The model under review builds one solid part; all positions refer to its coordinate system, in mm. A direction names the side the tool comes from. Coordinates: 2 decimals unless noted, no trailing zeros. Write each loop counter-clockwise with the first axis right and the second up, starting at its lowest first coordinate (ties: lowest second). Pieces come first, ordered by that corner, then holes. Notation, with made-up numbers: M 44,76 L 51,76 A12 cw 51,86 Z; hole C 48,52.25 d5. An arc over 180 degrees is marked long. Answer as CSV lines item,"result". Start each with the question number.
from build123d import *

# Parameters (mm, degrees)
F0_W        = 67.24
F0_H        = 39
F1_DEPTH    = 1.5
F2_T1_DEPTH = 49.2867319519
F3_T1_DEPTH = 73.5267319519
F3_T3_DEPTH = 43.5142834408
F4_R        = 1
F5_DEPTH    = 2
F6_W        = 16
F6_H        = 3.0143252599
F7_DEPTH    = 2


# Not quite as in the source:
# - a fillet or chamfer that OpenCascade refuses, or shapes differently, is made with other operations: its cross-section is extruded or revolved along the edge and cut away or added


with BuildPart() as f1:
    # F0 (on Top) → F1 (new body)
    with BuildSketch(Plane.XY):
        with Locations((12.5632099807, -23.9098862686)):
            Rectangle(F0_W, F0_H)
    extrude(amount=F1_DEPTH)

    # F2: chamfer of 2 on 2 edges, made by hand

    # F2_s2 → F2_t1 (cut)
    with BuildSketch(Plane.XZ.offset(-0.7334797074)):
        Polygon((46.1832099807, -0.5), (44.1832099807, 1.5), (46.1832099807, 1.5), align=None)
        Polygon((-21.0567900193, -0.5), (-19.0567900193, 1.5), (-21.0567900193, 1.5), align=None)
    extrude(amount=F2_T1_DEPTH, mode=Mode.SUBTRACT)

    # F3: chamfer of 2 on 4 edges, made by hand

    # F3_s2 → F3_t1 (cut)
    with BuildSketch(Plane.YZ.offset(-24.2001559952)):
        Polygon((-4.4098862686, -0.5), (-6.4098862686, 1.5), (-4.4098862686, 1.5), align=None)
        Polygon((-41.4098862686, 1.5), (-43.4098862686, -0.5), (-43.4098862686, 1.5), align=None)
    extrude(amount=F3_T1_DEPTH, mode=Mode.SUBTRACT)

    # F3_s4 → F3_t3 (cut)
    with BuildSketch(Plane.XZ.offset(2.1527445482)):
        Polygon((43.354782856, 1.5), (44.7689964183, 0.9142135624), (44.1832099807, 1.5), align=None)
        Polygon((-19.6425764569, 0.9142135624), (-18.2283628946, 1.5), (-19.0567900193, 1.5), align=None)
    extrude(amount=F3_T3_DEPTH, mode=Mode.SUBTRACT)

    # F4 (on face) → F5 (cut)
    with BuildSketch(Plane.XY.offset(1.5)):
        with Locations((43.1832099807, -40.4098862686)):
            Circle(F4_R)
        with Locations((43.1832099807, -7.4098862686)):
            Circle(F4_R)
        with Locations((-18.0567900193, -40.4098862686)):
            Circle(F4_R)
        with Locations((-18.0567900193, -7.4098862686)):
            Circle(F4_R)
    extrude(amount=-F5_DEPTH, mode=Mode.SUBTRACT)

    # F6 (on face) → F7 (cut)
    with BuildSketch(Plane.XY.offset(1.5)):
        with Locations((12.6832099807, -10.7027236386)):
            Rectangle(F6_W, F6_H)
    extrude(amount=-F7_DEPTH, mode=Mode.SUBTRACT)


solid = f1.part
1) Clearance check with flat-ended pins moving along their axes: pin 1 Ø0.8 at (x, z) = (9.5, 0.5) entering from -Y; pin 2 Ø2.5 at (x, y) = (-18.06, -40.41) entering from +Z. State where each tip first meets the part, or that it passes through.
2) To check wall thickness, follow line 1 (Y direction, x = 42.5, z = 0.15); line 2 (X direction, y = -7.5, z = 0.8); line 3 (X direction, y = -8, z = 0.5). State the ranges of each line that lie inside material, in increasing order. Write a range as [from, to].
3) Take a section at C-C on y = -24. Give the boundary of the cut face in (x, z).
4) Mouldability with a two-part tool opening along Y and no side actions: class faces 1 (the flat face through (-18.95, -23.66, 1.2)), 2 (the flat face through (12.1, -42.15, 0.76)), 3 (the cylindrical face through (-17.103, -7.11, 0.761)) as +Y half, -Y half, draft (parallel to the pull), parting line (faces both ways), or undercut.
5) Tool access review of faces 4 (the flat face through (12.1, -5.65, 0.74)), 5 (the flat face through (4.683, -11, 1)): name each direction out of +Z, -Z, +X, -X, +Y, -Y from which nothing blocks a thin tool from reaching the whole face with its end or side.
6) Take a section at B-B on z = 0.5. Give the boundary of the cut face in (x, y).
7) Take a section at A-A on x = 10. Give the boundary of the cut face in (y, z).
8) Take a section at D-D on x = 22. Give the boundary of the cut face in (y, z), and give its area (4 significant figures).
Results:
1,pin 1,"stops at y = -42.81"
1,pin 2,"stops at z = 1.5"
2,line 1,"y = [-42.76, -41.14], [-39.68, -8.14], [-6.68, -5.06]"
2,line 2,"x = [-19.76, -19.05], [-17.06, 42.19], [44.18, 44.88]"
2,line 3,"x = [-20.06, -18.86], [-17.25, 42.38], [43.99, 45.18]"
3,outline,"M -20.56,0 L 45.68,0 L 44.77,0.91 L 43.35,1.5 L -18.23,1.5 L -19.64,0.91 Z"
4,face 1,"draft"
4,face 2,"-Y half"
4,face 3,"undercut"
5,face 4,"+Z, +X, -X, +Y"
5,face 5,"+Z, -Z"
6,outline,"M -20.06,-42.41 L 45.18,-42.41 L 45.18,-5.41 L -20.06,-5.41 Z; hole C -18.06,-40.41 d2; hole C -18.06,-7.41 d2; hole M 4.68,-12.21 L 20.68,-12.21 L 20.68,-9.2 L 4.68,-9.2 Z; hole C 43.18,-40.41 d2; hole C 43.18,-7.41 d2"
7,outline,"M -42.91,0 L -12.21,0 L -12.21,1.5 L -41.41,1.5 Z; M -9.2,0 L -4.91,0 L -6.41,1.5 L -9.2,1.5 Z"
8,outline,"M -42.91,0 L -4.91,0 L -6.41,1.5 L -41.41,1.5 Z"
8,area,"54.75 mm²"
